```python
from build123d import *

# Parameters (mm, degrees)
BOSS_EXTRUDE2_DEPTH = 63.5
SKETCH1_4_W         = 13.909610768
SKETCH1_4_H         = 11.124423297
BOSS_EXTRUDE3_DEPTH = 5.08
SKETCH2_R           = 3.175
CUT_EXTRUDE1_DEPTH  = 2.54
SKETCH3_R           = 1.905
CUT_EXTRUDE2_DEPTH  = 94.48175649
CUT_EXTRUDE3_START  = -43.382423
SKETCH4_R           = 13.208
CUT_EXTRUDE3_DEPTH  = 17.272
FILLET1_R           = 5.08


with BuildPart() as part:
    # Sketch1 → Boss-Extrude2 (new body)
    with BuildSketch(Plane(origin=(0, 0, 0), x_dir=(1, 0, 0), z_dir=(0, 1, 0))):
        with BuildLine():
            ThreePointArc((0, 63.287802336), (-16.535030554, 61.029206749), (-31.896257962, 54.506846594))
            Line((-31.896257962, 54.506846594), (-31.896257962, 43.382423297))
            Line((-31.896257962, 43.382423297), (-17.986647194, 43.382423297))
            ThreePointArc((-17.986647194, 43.382423297), (-9.699677374, 48.846444583), (0, 50.954917077))
            ThreePointArc((0, 50.954917077), (9.699677374, 48.846444583), (17.986647194, 43.382423297))
            Line((17.986647194, 43.382423297), (31.896257962, 43.382423297))
            Line((31.896257962, 43.382423297), (31.896257962, 54.506846594))
            ThreePointArc((31.896257962, 54.506846594), (16.535030554, 61.029206749), (0, 63.287802336))
        make_face()
    extrude(amount=BOSS_EXTRUDE2_DEPTH)

    # Sketch1<4> → Boss-Extrude3 (add)
    with BuildSketch(Plane(origin=(0, 0, 0), x_dir=(1, 0, 0), z_dir=(0, 1, 0))):
        with Locations((-24.941452578, 37.820211649)):
            Rectangle(SKETCH1_4_W, SKETCH1_4_H)
        with Locations((24.941452578, 37.820211649)):
            Rectangle(SKETCH1_4_W, SKETCH1_4_H)
    extrude(amount=BOSS_EXTRUDE3_DEPTH)

    # Sketch2 → Cut-Extrude1 (cut)
    with BuildSketch(Plane(origin=(0, 5.08, 0), x_dir=(1, 0, 0), z_dir=(0, 1, 0))):
        with Locations(Location((-24.941452578, 37.820211648, 0), (0, 0, 270))):
            Circle(SKETCH2_R)
        with Locations(Location((24.941452578, 37.820211648, 0), (0, 0, 90))):
            Circle(SKETCH2_R)
    extrude(amount=-CUT_EXTRUDE1_DEPTH, mode=Mode.SUBTRACT)

    # Sketch3 → Cut-Extrude2 (cut, through all)
    with BuildSketch(Plane(origin=(0, 2.54, 0), x_dir=(1, 0, 0), z_dir=(0, 1, 0))):
        with Locations(Location((-24.941452578, 37.820211648, 0), (0, 0, 270))):
            Circle(SKETCH3_R)
        with Locations(Location((24.941452578, 37.820211648, 0), (0, 0, 90))):
            Circle(SKETCH3_R)
    extrude(amount=-CUT_EXTRUDE2_DEPTH, mode=Mode.SUBTRACT)

    # Sketch4 → Cut-Extrude3 (cut)
    with BuildSketch(Plane.XY.offset(CUT_EXTRUDE3_START)):
        with Locations((0, 26.175500537)):
            Circle(SKETCH4_R)
    extrude(amount=-CUT_EXTRUDE3_DEPTH, mode=Mode.SUBTRACT)

    # Fillet1
    fillet1_edges = [part.edges().sort_by_distance(p)[0] for p in [
        (31.896257962, 31.75, -54.506846594),
        (-31.896257962, 31.75, -54.506846594),
    ]]
    fillet(fillet1_edges, radius=FILLET1_R)


solid = part.part
```
Input: part model. Units: mm. Frame: model coordinates. A direction names the side the tool comes from. Coordinates: 2 decimals unless noted, no trailing zeros. Loops run counter-clockwise (first coordinate to the right, second up) from the corner with the lowest first, then second, coordinate; pieces in that order, holes last. Notation, with made-up numbers: (-15, -13.75) - (6, -13.75) arc R23 ccw to (6, 5.25) - close; hole circle Ø3 at (1, 66.25). An arc over 180 degrees is marked (long way). Answer in a Markdown table with one row per item.
(1) Material intervals for L1, parallel to Y at x = 0, z = -51; L2, parallel to X at y = 58.5, z = -47; L3, parallel to Z at x = 0, y = 36, sorted ascending. Write a range as from..to.
Model answer:
| item | result |
|---|---|
| L1 | y = 0..12.97, 39.38..63.5 |
| L2 | x = -31.9..-13.3, 13.3..31.9 |
| L3 | z = -63.29..-60.65 |
(2) Set-up query: faces 4 (the face through (13.511, 31.306, -46.872)), 5 (the face through (-28.1, 5.08, -39.1)), 6 (the face through (0, 26, -60.654)), 7 (the face through (-24.802, 3.828, -40.992)). Return all of +Z, -Z, +X, -X, +Y, -Y with unobstructed straight access to the full face (end or side cutting, diameter ignored); none if empty.
Model answer:
| item | result |
|---|---|
| face 4 | +Z, +Y, -Y |
| face 5 | +Z, +X, -X, +Y |
| face 6 | +Z |
| face 7 | +Y |
(3) Pin query (flat end, axial travel): P1, Ø5.5, axis at x = -28.5, z = -36.5, coming from the +Y side; P2, Ø1, axis at y = 30, z = -52.5, coming from the -X side; P3, Ø5, axis at x = 21.5, y = 42, coming from the -Z side. Return the tip coordinate at first contact, or that it passes through.
Model answer:
| item | result |
|---|---|
| P1 | stops at y = 5.08 |
| P2 | stops at x = -31.87 |
| P3 | stops at z = -60.3 |
(4) Mould query, pull axis X, two halves, no side actions, for faces 1 (the face through (-26, 2.54, -36)), 2 (the face through (25, 3, -32.258)), 3 (the face through (-31.186, 32.194, -54.12)). Classes: pulls with the +X half, pulls with the -X half, needs draft (parallel to the pull), parting line crosses it, or undercut.
Model answer:
| item | result |
|---|---|
| face 1 | undercut |
| face 2 | needs draft |
| face 3 | pulls with the -X half |
(5) Cut plane D-D on z = -45. Output: boundary loops of the cut face in (x, y), plus the area to 3 significant figures.
Model answer:
| item | result |
|---|---|
| outline | (-31.9, 0) - (-16.15, 0) - (-16.15, 63.5) - (-31.9, 63.5) - close; (16.15, 0) - (31.9, 0) - (31.9, 63.5) - (16.15, 63.5) - close |
| area | 2,000 mm² |
(6) Cut plane A-A on y = 7.5. Output: boundary loops of the cut face in (x, z).
Model answer:
| item | result |
|---|---|
| outline | (-31.9, -51.53) arc R5.08 ccw to (-29.19, -56.02) arc R62.98 ccw to (0, -63.29) arc R62.98 ccw to (29.19, -56.02) arc R5.08 ccw to (31.9, -51.53) - (31.9, -43.38) - (17.99, -43.38) arc R27.06 cw to (0, -50.95) arc R27.06 cw to (-17.99, -43.38) - (-31.9, -43.38) - close |
(7) Cut plane B-B on z = -49.5. Output: boundary loops of the cut face in (x, y).
Model answer:
| item | result |
|---|---|
| outline | (-31.9, 0) - (-7.99, 0) - (-7.99, 15.66) arc R13.21 cw to (-7.99, 36.69) - (-7.99, 63.5) - (-31.9, 63.5) - close; (7.99, 0) - (31.9, 0) - (31.9, 63.5) - (7.99, 63.5) - (7.99, 36.69) arc R13.21 cw to (7.99, 15.66) - close |
(8) Cut plane C-C on x = -20.5. Output: boundary loops of the cut face in (y, z), plus the area to 3 significant figures.
Model answer:
| item | result |
|---|---|
| outline | (0, -59.8) - (63.5, -59.8) - (63.5, -43.38) - (5.08, -43.38) - (5.08, -32.26) - (0, -32.26) - close |
| area | 1,100 mm² |
